```python
from build123d import *

# Parameters (mm, degrees)
BOSS_EXTRUDE1_DEPTH = 2.794
BOSS_EXTRUDE2_DEPTH = 7.62


with BuildPart() as part:
    # Sketch1 → Boss-Extrude1 (new body)
    with BuildSketch(Plane(origin=(0, 0, 0), x_dir=(1, 0, 0), z_dir=(0, 1, 0))):
        Polygon((7.62, 25.4), (5.715, 25.4), (5.715, 5.715), (25.4, 5.715), (25.4, 7.62), (7.62, 7.62), align=None)
        Polygon((5.715, 25.4), (1.905, 25.4), (1.905, 1.905), (25.4, 1.905), (25.4, 5.715), (5.715, 5.715), align=None)
        Polygon((0, 25.4), (0, 0), (25.4, 0), (25.4, 1.905), (1.905, 1.905), (1.905, 25.4), align=None)
    extrude(amount=BOSS_EXTRUDE1_DEPTH)

    # Sketch1_6 → Boss-Extrude2 (add)
    with BuildSketch(Plane(origin=(0, 0, 0), x_dir=(1, 0, 0), z_dir=(0, 1, 0))):
        Polygon((0, 25.4), (0, 0), (25.4, 0), (25.4, 1.905), (1.905, 1.905), (1.905, 25.4), align=None)
        Polygon((7.62, 25.4), (5.715, 25.4), (5.715, 5.715), (25.4, 5.715), (25.4, 7.62), (7.62, 7.62), align=None)
    extrude(amount=-BOSS_EXTRUDE2_DEPTH)


solid = part.part
```
For this review, take the finished solid that the model builds, in its own axes (mm). A direction names the side the tool comes from. Round coordinates to 2 decimals unless told otherwise and drop trailing zeros. Order: outer loops, then holes, each group sorted by start corner. A loop starts at its lowest first (then second) coordinate and runs counter-clockwise, first axis right, second up.
Q1. We need section B-B, the plane x = 9.25. Give the boundary of the cut face in (y, z) (3 decimals), plus the area to 3 significant figures.
Findings below:
outline: (-7.62, -7.62) - (2.794, -7.62) - (2.794, 0) - (-7.62, 0) - (-7.62, -1.905) - (0, -1.905) - (0, -5.715) - (-7.62, -5.715) - close
area: 50.3 mm2
Q2. Wall thickness on line 1 (Z direction, x = 14.75, y = -6.75) (3 decimals); line 2 (X direction, y = -3, z = -9.75) (3 decimals); line 3 (X direction, y = 0.25, z = -12.25): over which ranges is each line inside the solid? List them lowest first.
Findings below:
line 1: z = -7.62 to -5.715, -1.905 to 0
line 2: x = 0 to 1.905, 5.715 to 7.62
line 3: x = 0 to 7.62
Q3. Mouldability with a two-part tool opening along Z and no side actions: class faces 5 (the flat face through (14, -4, -1.905)), 6 (the flat face through (13, -2, 0)), 7 (the flat face through (1, -7.62, -7)), 8 (the flat face through (17, -2, -7.62)) as pulls with the +Z half, pulls with the -Z half, needs draft (parallel to the pull), parting line crosses it, or undercut.
Findings below:
face 5: undercut
face 6: pulls with the +Z half
face 7: needs draft
face 8: pulls with the -Z half
Q4. We need section D-D, the plane y = 1.5. Give the boundary of the cut face in (x, z), plus the area to 3 significant figures.
Findings below:
outline: (0, -25.4) - (7.62, -25.4) - (7.62, -7.62) - (25.4, -7.62) - (25.4, 0) - (0, 0) - close
area: 329 mm2
Q5. We need section C-C, the plane z = -4.5. Give the boundary of the cut face in (x, y) (3 decimals).
Findings below:
outline: (0, -7.62) - (1.905, -7.62) - (1.905, 0) - (25.4, 0) - (25.4, 2.794) - (0, 2.794) - close
Q6. Machinability: for faces 1 (the flat face through (7.62, -2, -16)), 2 (the flat face through (7, -7.62, -11)), 3 (the flat face through (15, -4, -5.715)), 4 (the flat face through (5.715, -4, -16)), which of the approach directions +Z, -Z, +X, -X, +Y, -Y give a long, thin tool a straight path to every point of the face, cutting with its end or side? Answer none if there is none.
Findings below:
face 1: -Z, +X, +Y, -Y
face 2: +Z, -Z, +X, -X, -Y
face 3: +X, -Y
face 4: -Z, -Y
Q7. We need section A-A, the plane y = -3.25. Give the boundary of the cut face in (x, z) (3 decimals), plus the area to 3 significant figures.
Findings below:
outline: (0, -25.4) - (1.905, -25.4) - (1.905, -1.905) - (25.4, -1.905) - (25.4, 0) - (0, 0) - close; (5.715, -25.4) - (7.62, -25.4) - (7.62, -7.62) - (25.4, -7.62) - (25.4, -5.715) - (5.715, -5.715) - close
area: 165 mm2
Q8. Insertion check: P1, Ø6, axis at y = -5.5, z = -11.5, coming from the -X side; P2, Ø6, axis at x = 13, y = -2.5, coming from the -Z side; P3, Ø4, axis at y = -2.5, z = -16, coming from the +X side. Each pin has a flat end and moves straight along its axis. Give the tip position at first contact, or say it passes through.
Findings below:
P1: stops at x = 0
P2: stops at z = -7.62
P3: stops at x = 7.62
